The listing builds one solid part. Answer for the finished solid, in the listing's coordinates (mm). A direction names the side the tool comes from. Coordinates: 2 decimals unless noted, no trailing zeros. Loops run counter-clockwise (first coordinate to the right, second up) from the corner with the lowest first, then second, coordinate; pieces in that order, holes last. Notation, with made-up numbers: (68.5, -35) - (79.5, -35) arc R37 cw to (79.5, 2) - close; hole circle Ø6 at (-17, -5). An arc over 180 degrees is marked (long way). Return JSON: item names as keys, results as strings. Group by question number.
1. Which of the six approach directions +Z, -Z, +X, -X, +Y, -Y give full straight-line access (tool end or side, diameter ignored) to faces 1 (the face through (-4, 30, -4)), 2 (the face through (315, 38.608, 73)), 3 (the face through (-315, 75, 4))?
2. This flat-tipped pin is pushed along its axis until it touches: P1, Ø12, axis at x = 85, z = 124.5, coming from the +Y side. Where does it stop, or does it pass through?
3. Section B-B (x = -146) is taken. Write down the section's boundary in (y, z).
4. Section A-A (z = 101.5) is taken. State how many separate pieces and enclosed holes the cut face has, and give its area (3 significant figures).
5. Find the intervals of material crossed by line 1 along X through (y, z) = (64, 268); line 2 along Y through (x, z) = (-168, 77.5); line 3 along X through (y, z) = (37, -117), in increasing order.
6. The mould has two halves that part along Z. Classify faces 4 (the face through (-315, 68.608, 78)), 5 (the face through (5, 12, 300)), 6 (the face through (-300, 69, 4)): pulls with the +Z half, pulls with the -Z half, needs draft (parallel to the pull), parting line crosses it, or undercut.
```python
from build123d import *

# Parameters (mm, degrees)
SKETCH1_W           = 600
SKETCH1_H           = 600
BOSS_EXTRUDE1_DEPTH = 30
SKETCH2_W           = 600
SKETCH2_H           = 75
SKETCH2_R           = 15
BOSS_EXTRUDE2_DEPTH = 30
CUT_EXTRUDE4_START  = -631
CUT_EXTRUDE4_DEPTH  = 661
FILLET1_R           = 10


with BuildPart() as part:
    # Sketch1 → Boss-Extrude1 (new body)
    with BuildSketch(Plane(origin=(0, 0, 0), x_dir=(1, 0, 0), z_dir=(0, 1, 0))):
        Rectangle(SKETCH1_W, SKETCH1_H)
    extrude(amount=BOSS_EXTRUDE1_DEPTH)

    # Sketch2 → Boss-Extrude2 (add)
    with BuildSketch(Plane(origin=(300, 0, 0), x_dir=(0, 0, -1), z_dir=(1, 0, 0))):
        with Locations((0, 37.5)):
            Rectangle(SKETCH2_W, SKETCH2_H)
        with Locations((258.993384408, 53.607709477)):
            Circle(SKETCH2_R, mode=Mode.SUBTRACT)
    boss_extrude2 = extrude(amount=BOSS_EXTRUDE2_DEPTH)

    # Sketch3 → Cut-Extrude4 (cut)
    with BuildSketch(Plane(origin=(330, 0, 0), x_dir=(0, 0, -1), z_dir=(1, 0, 0)).offset(CUT_EXTRUDE4_START)):
        with BuildLine():
            Line((-250, 68.607709477), (99.736599438, 68.607709477))
            ThreePointArc((99.736599438, 68.607709477), (114.736599438, 53.607709477), (99.736599438, 38.607709477))
            Line((99.736599438, 38.607709477), (-250, 38.607709477))
            ThreePointArc((-250, 38.607709477), (-265, 53.607709477), (-250, 68.607709477))
        make_face()
    cut_extrude4 = extrude(amount=CUT_EXTRUDE4_DEPTH, mode=Mode.SUBTRACT)

    # Mirror1: Boss-Extrude2, Cut-Extrude4 across plane
    add(boss_extrude2.mirror(Plane(origin=(0, 0, 0), x_dir=(0, 0, 1), z_dir=(1, 0, 0))))
    add(cut_extrude4.mirror(Plane(origin=(0, 0, 0), x_dir=(0, 0, 1), z_dir=(1, 0, 0))), mode=Mode.SUBTRACT)

    # Fillet1
    fillet1_edges = [part.edges().sort_by_distance(p)[0] for p in [
        (300, 30, 0),
        (-300, 30, 0),
    ]]
    fillet(fillet1_edges, radius=FILLET1_R)


solid = part.part
```
The answers:
{
 "1": {"face 1": "+Z, -Z, +Y", "face 2": "+X, -X", "face 3": "+Z, -Z, +X, -X, +Y"},
 "2": {"P1": "stops at y = 30"},
 "3": {"outline": "(0, -300) - (30, -300) - (30, 300) - (0, 300) - close"},
 "4": {"separate pieces": "3", "enclosed holes": "0", "area": "20,700 mm2"},
 "5": {"line 1": "x = -330 to -300, 300 to 330", "line 2": "y = 0 to 30", "line 3": "x = -330 to -299.54, 299.54 to 330"},
 "6": {"face 4": "undercut", "face 5": "pulls with the +Z half", "face 6": "needs draft"}
}
